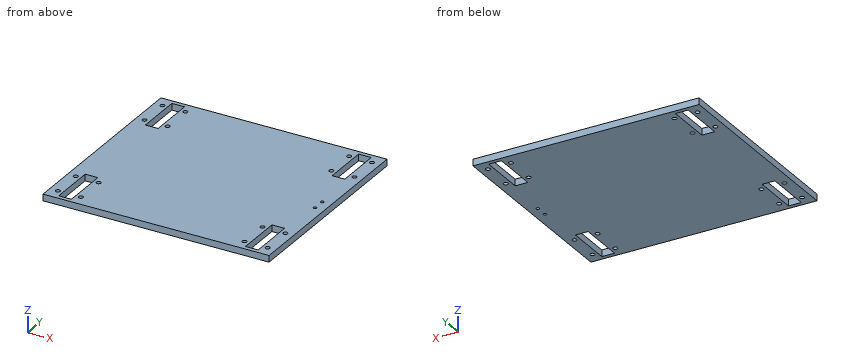
```python
from build123d import *

# Parameters (mm, degrees)
F0_W     = 175.01715
F0_H     = 158.2801
F0_R     = 1.7272
F0_W_2   = 9.8425
F0_H_2   = 35.56
F0_R_2   = 1.25
F1_DEPTH = 5.08


with BuildPart() as f1:
    # F0 (on Top) → F1 (new body)
    with BuildSketch(Plane.XY):
        Rectangle(F0_W, F0_H)
        with Locations((-81.158575, -70.12305)):
            Circle(F0_R, mode=Mode.SUBTRACT)
        with Locations((-63.378575, -70.12305)):
            Circle(F0_R, mode=Mode.SUBTRACT)
        with Locations((-72.268575, -58.18505)):
            Rectangle(F0_W_2, F0_H_2, mode=Mode.SUBTRACT)
        with Locations((-81.158575, -46.24705)):
            Circle(F0_R, mode=Mode.SUBTRACT)
        with Locations((-63.378575, -46.24705)):
            Circle(F0_R, mode=Mode.SUBTRACT)
        with Locations((63.378575, -70.12305)):
            Circle(F0_R, mode=Mode.SUBTRACT)
        with Locations((81.158575, -70.12305)):
            Circle(F0_R, mode=Mode.SUBTRACT)
        with Locations((63.378575, -46.24705)):
            Circle(F0_R, mode=Mode.SUBTRACT)
        with Locations((72.268575, -58.18505)):
            Rectangle(F0_W_2, F0_H_2, mode=Mode.SUBTRACT)
        with Locations((81.158575, -46.24705)):
            Circle(F0_R, mode=Mode.SUBTRACT)
        with Locations((80.208564, -4.750003)):
            Circle(F0_R_2, mode=Mode.SUBTRACT)
        with Locations((-81.158575, 46.24705)):
            Circle(F0_R, mode=Mode.SUBTRACT)
        with Locations((-72.268575, 58.18505)):
            Rectangle(F0_W_2, F0_H_2, mode=Mode.SUBTRACT)
        with Locations((-63.378575, 46.24705)):
            Circle(F0_R, mode=Mode.SUBTRACT)
        with Locations((-81.158575, 70.12305)):
            Circle(F0_R, mode=Mode.SUBTRACT)
        with Locations((-63.378575, 70.12305)):
            Circle(F0_R, mode=Mode.SUBTRACT)
        with Locations((80.208564, 4.750003)):
            Circle(F0_R_2, mode=Mode.SUBTRACT)
        with Locations((63.378575, 46.24705)):
            Circle(F0_R, mode=Mode.SUBTRACT)
        with Locations((81.158575, 46.24705)):
            Circle(F0_R, mode=Mode.SUBTRACT)
        with Locations((72.268575, 58.18505)):
            Rectangle(F0_W_2, F0_H_2, mode=Mode.SUBTRACT)
        with Locations((63.378575, 70.12305)):
            Circle(F0_R, mode=Mode.SUBTRACT)
        with Locations((81.158575, 70.12305)):
            Circle(F0_R, mode=Mode.SUBTRACT)
    extrude(amount=F1_DEPTH)


solid = f1.part
```
Here's how the part is built. I have some questions about the finished solid (model axes, mm). Round coordinates to 2 decimals unless told otherwise and drop trailing zeros. Order: outer loops, then holes, each group sorted by start corner. A loop starts at its lowest first (then second) coordinate and runs counter-clockwise, first axis right, second up. Notation, with made-up numbers: M -16,12.5 L 11,12.5 A13 cw 11,30.5 Z; hole C 17.25,56 d5. An arc over 180 degrees is marked long. Use CSV: the item, a comma, the result in double quotes.
1) I want a section at B-B (x = 74). List the corners of the cut face in (y, z) for me.
Taken from the geometry:
outline,"M -79.14,0 L -75.97,0 L -75.97,5.08 L -79.14,5.08 Z; M -40.41,0 L 40.41,0 L 40.41,5.08 L -40.41,5.08 Z; M 75.97,0 L 79.14,0 L 79.14,5.08 L 75.97,5.08 Z"
2) I'm going to push flat-ended pins straight in: P1, Ø2, axis at x = -63.38, y = -70.12, coming from the -Z side; P2, Ø6, axis at x = 36.5, y = -44.5, coming from the -Z side. Where does each tip first touch, or does it pass through?
Taken from the geometry:
P1,"through"
P2,"z = 0"
3) I want a section at A-A (y = 66). List the corners of the cut face in (x, z) for me, then the cut area to 3 significant figures.
Taken from the geometry:
outline,"M -87.51,0 L -77.19,0 L -77.19,5.08 L -87.51,5.08 Z; M -67.35,0 L 67.35,0 L 67.35,5.08 L -67.35,5.08 Z; M 77.19,0 L 87.51,0 L 87.51,5.08 L 77.19,5.08 Z"
area,"789 mm^2"
4) I want a section at C-C (z = 1.3). Count the separate pieces of the cut face and the enclosed holes in it, then the cut area to 3 significant figures.
Taken from the geometry:
separate pieces,"1"
enclosed holes,"22"
area,"26,100 mm^2"
5) I need wall thicknesses on line 1 along X through (y, z) = (52, 1.65). Which ranges of the line are inside material? Lowest first, please. Write a range as [from, to].
Taken from the geometry:
line 1,"[-87.51, -77.19], [-67.35, 67.35], [77.19, 87.51]"
